```python
from build123d import *

# Parameters (mm, degrees)
SKETCH1_W             = 42
SKETCH1_H             = 7
SKETCH1_R             = 1.5
BOSS_EXTRUDE1_DEPTH   = 12
SKETCH1_H_2           = 6.75
BOSS_EXTRUDE1_2_DEPTH = 12
SKETCH2_R             = 1.5
BOSS_EXTRUDE2_DEPTH   = 5
SKETCH2_3_W           = 6
SKETCH2_3_H           = 26.85
BOSS_EXTRUDE3_DEPTH   = 5
BOSS_EXTRUDE4_START   = 12
SKETCH1_3_W           = 42
SKETCH1_3_H           = 13.25
BOSS_EXTRUDE4_DEPTH   = 3


with BuildPart() as part:
    # Sketch1 → Boss-Extrude1 (new body)
    with BuildSketch(Plane.XY):
        with Locations((0, -10)):
            Rectangle(SKETCH1_W, SKETCH1_H)
        with Locations((-10, -10)):
            Circle(SKETCH1_R, mode=Mode.SUBTRACT)
        with Locations((10, -10)):
            Circle(SKETCH1_R, mode=Mode.SUBTRACT)
    extrude(amount=BOSS_EXTRUDE1_DEPTH)

    # Sketch2 → Boss-Extrude2 (add)
    with BuildSketch(Plane.XZ.offset(13.5)):
        Polygon((21, 12), (-21, 12), (-21, -37), (-2.5, -37), (-2.5, -49), (2.5, -49), (2.5, -37), (21, -37), align=None)
        with Locations((-8.5, -34)):
            Circle(SKETCH2_R, mode=Mode.SUBTRACT)
        with Locations((8.5, -34)):
            Circle(SKETCH2_R, mode=Mode.SUBTRACT)
        with Locations((0, -46)):
            Circle(SKETCH2_R, mode=Mode.SUBTRACT)
    extrude(amount=BOSS_EXTRUDE2_DEPTH)

    # Sketch2<3> → Boss-Extrude3 (add)
    with BuildSketch(Plane.XZ.offset(13.5)):
        with Locations((18, -23.575)):
            Rectangle(SKETCH2_3_W, SKETCH2_3_H)
        with Locations((-18, -23.575)):
            Rectangle(SKETCH2_3_W, SKETCH2_3_H)
    extrude(amount=-BOSS_EXTRUDE3_DEPTH)



with BuildPart() as body_2:
    # Sketch1 → Boss-Extrude1 2 (new body)
    with BuildSketch(Plane.XY):
        with Locations((0, 10.125)):
            Rectangle(SKETCH1_W, SKETCH1_H_2)
        with Locations((10, 10)):
            Circle(SKETCH1_R, mode=Mode.SUBTRACT)
        with Locations((-10, 10)):
            Circle(SKETCH1_R, mode=Mode.SUBTRACT)
    extrude(amount=BOSS_EXTRUDE1_2_DEPTH)


with BuildPart() as part_1:
    add(part.part)

    add(body_2.part)  # Boss-Extrude4 merges body 2
    # Sketch1<3> → Boss-Extrude4 (add)
    with BuildSketch(Plane.XY.offset(BOSS_EXTRUDE4_START)):
        with Locations((0, 0.125)):
            Rectangle(SKETCH1_3_W, SKETCH1_3_H)
    extrude(amount=-BOSS_EXTRUDE4_DEPTH)


solid = part_1.part
```
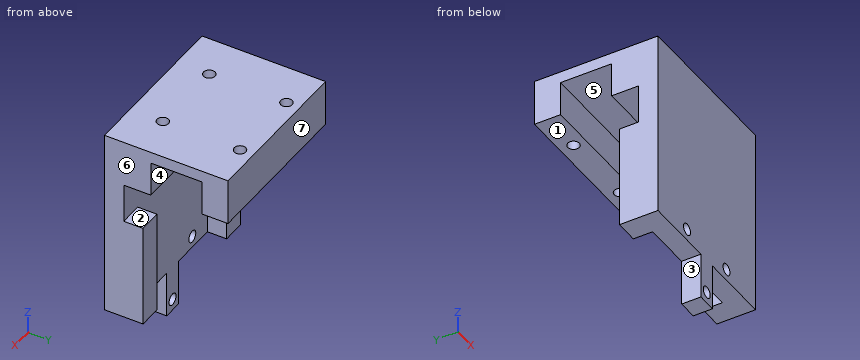
For this review, take the finished solid that the model builds, in its own axes (mm). Face numbers are marked on the shaded views. A direction names the side the tool comes from. Coordinates: 2 decimals unless noted, no trailing zeros. Loops run counter-clockwise (first coordinate to the right, second up) from the corner with the lowest first, then second, coordinate; pieces in that order, holes last. Notation, with made-up numbers: (34, 15.5) -> (52, 15.5) arc R27 cw to (52, 49.5) -> close; hole circle Ø8 at (58.25, 83.25). An arc over 180 degrees is marked (long way). Return JSON: item names as keys, results as strings. Group by question number.
(1) Consider section B-B, the plane x = 0. Give the boundary of the cut face in (y, z).
(2) Tool access review of the marked faces 1, 2 and 3: name each direction out of +Z, -Z, +X, -X, +Y, -Y from which nothing blocks a thin tool from reaching the whole face with its end or side.
(3) To check wall thickness, follow L1, parallel to Y at x = 10, z = 3; L2, parallel to X at y = -10, z = -13.5; L3, parallel to X at y = -16.5, z = -34.5. State the ranges of each line that lie inside material, in increasing order.
(4) For pin 1 Ø1.8 at (x, z) = (0, -46) entering from -Y; pin 2 Ø3.5 at (x, y) = (-0.5, 10.5) entering from -Z; pin 3 Ø1.5 at (x, y) = (16, -8) entering from -Z; pin 4 Ø6.5 at (x, y) = (-7, -3) entering from -Z, all flat-tipped, find the tip position at first contact; note any pin that passes through.
(5) Mouldability with a two-part tool opening along Y and no side actions: class the marked faces 4, 5, 6 and 7 as pulls with the +Y half, pulls with the -Y half, needs draft (parallel to the pull), parting line crosses it, or undercut.
(6) Consider section C-C, the plane y = -10. Give the boundary of the cut face in (x, z).
(7) Consider section A-A, the plane z = 3.5. Give the boundary of the cut face in (x, y).
(8) Consider section D-D, the plane z = -34. Give the boundary of the cut face in (x, y).
Results below:
{
 "1": {"outline": "(-18.5, -49) -> (-13.5, -49) -> (-13.5, -47.5) -> (-18.5, -47.5) -> close; (-18.5, -44.5) -> (-13.5, -44.5) -> (-13.5, 0) -> (-6.5, 0) -> (-6.5, 9) -> (6.75, 9) -> (6.75, 0) -> (13.5, 0) -> (13.5, 12) -> (-18.5, 12) -> close"},
 "2": {"face 1": "-Z, +X, -X, +Y", "face 2": "+X, -X, +Y", "face 3": "-Z, -X, +Y, -Y"},
 "3": {"L1": "y = -18.5 to -11.5, -8.5 to -6.5, 6.75 to 8.5, 11.5 to 13.5", "L2": "x = -21 to -15, 15 to 21", "L3": "x = -21 to -9.91, -7.09 to 7.09, 9.91 to 21"},
 "4": {"pin 1": "passes through", "pin 2": "stops at z = 0", "pin 3": "stops at z = -37", "pin 4": "stops at z = 9"},
 "5": {"face 4": "undercut", "face 5": "undercut", "face 6": "needs draft", "face 7": "pulls with the +Y half"},
 "6": {"outline": "(-21, -37) -> (-15, -37) -> (-15, -10.15) -> (-21, -10.15) -> close; (-21, 0) -> (-11.5, 0) -> (-11.5, 12) -> (-21, 12) -> close; (-8.5, 0) -> (8.5, 0) -> (8.5, 12) -> (-8.5, 12) -> close; (11.5, 0) -> (21, 0) -> (21, 12) -> (11.5, 12) -> close; (15, -37) -> (21, -37) -> (21, -10.15) -> (15, -10.15) -> close"},
 "7": {"outline": "(-21, -18.5) -> (21, -18.5) -> (21, -6.5) -> (-21, -6.5) -> close; (-21, 6.75) -> (21, 6.75) -> (21, 13.5) -> (-21, 13.5) -> close; hole circle Ø3 at (-10, -10); hole circle Ø3 at (-10, 10); hole circle Ø3 at (10, -10); hole circle Ø3 at (10, 10)"},
 "8": {"outline": "(-21, -18.5) -> (-10, -18.5) -> (-10, -13.5) -> (-15, -13.5) -> (-15, -8.5) -> (-21, -8.5) -> close; (-7, -18.5) -> (7, -18.5) -> (7, -13.5) -> (-7, -13.5) -> close; (10, -18.5) -> (21, -18.5) -> (21, -8.5) -> (15, -8.5) -> (15, -13.5) -> (10, -13.5) -> close"}
}
